Verification items for the finished model (mm, model axes). Face numbers are marked on the shaded views. Round coordinates to 2 decimals unless told otherwise and drop trailing zeros. Write each loop counter-clockwise with the first axis right and the second up, starting at its lowest first coordinate (ties: lowest second). Pieces come first, ordered by that corner, then holes. Notation, with made-up numbers: M 23.25,86 L 34.25,86 A14 ccw 34.25,105 Z; hole C 37.5,23.25 d10. An arc over 180 degrees is marked long. One line per item, written item: value. Start each with the question number.
Item 1: Gauge pin test, flat ends, axial feed: pin 1 (0.9 mm diameter, centred on y = 1.5, z = -32, fed in from +X); pin 2 (1.5 mm diameter, centred on y = 2, z = -28, fed in from -X); pin 3 (1 mm diameter, centred on y = 2.5, z = -56.5, fed in from +X). Record the tip position at first contact, or that the pin passes through.
Item 2: Section check D-D, the plane x = -50.5. Record the cut outline in (y, z), then the cut area to 3 significant figures.
Item 3: Draft check along X on the marked faces 1 and 2. Enter one of: +X half, -X half, draft (parallel to the pull), parting line (faces both ways), or undercut.
Item 4: Section check A-A, the plane z = -54. Record the cut outline in (x, y).
Item 5: Thickness scan on probe 1 along Z at (x, y) = (-4, 2.55); probe 2 along Y at (x, z) = (-83, -25); probe 3 along X at (y, z) = (1.35, -63). Record the ranges inside material, lowest first. Write a range as from..to.
Item 6: Section check B-B, the plane x = -5. Record the cut outline in (y, z).
from build123d import *

# Parameters (mm, degrees)
P_IDAT_VYSUNUT_M1_DEPTH = 3
P_IDAT_VYSUNUT_M2_DEPTH = 2
ZAOBLIT3_R              = 1


with BuildPart() as part:
    # Skica1 → P_idat vysunut_m1 (new body)
    with BuildSketch(Plane(origin=(0, 0, 0), x_dir=(1, 0, 0), z_dir=(0, 1, 0))):
        Polygon((-118.143750166, 15), (-118.143750166, 0), (-102.227105248, 19.278496169), (-95.473037065, 43.348863075), (-82.997228437, 47.003202833), (-48.112980408, 27.430537213), (-19, 0), (0, 0), (0, 15), (9.950504516, 11.37831254), (9.950504516, 24.27831254), (-10.5, 24.27831254), (-10.5, 37.37831254), (0, 33.55662508), (0, 69.224902673), (-39.317553332, 46.524902673), (-78.635106664, 69.224902673), (-118.143185584, 46.414902673), (-118.143185584, 33.5570142), (-107.643750166, 37.378496169), (-107.643750166, 24.278496169), (-128.093750166, 24.278496169), (-128.093750166, 11.378496169), align=None)
    extrude(amount=P_IDAT_VYSUNUT_M1_DEPTH)

    # Skica1_3 → P_idat vysunut_m2 (add)
    with BuildSketch(Plane(origin=(0, 0, 0), x_dir=(1, 0, 0), z_dir=(0, 1, 0))):
        Polygon((-102.227105248, 19.278496169), (-118.143750166, 0), (-19, 0), (-48.112980408, 27.430537213), (-82.997228437, 47.003202833), (-95.473037065, 43.348863075), align=None)
    extrude(amount=P_IDAT_VYSUNUT_M2_DEPTH)

    # Zaoblit3
    zaoblit3_edges = [part.edges().sort_by_distance(p)[0] for p in [
        (-10.5, 1.5, -24.27831254),
        (9.950504516, 1.5, -24.27831254),
        (9.950504516, 1.5, -11.37831254),
        (0, 1.5, -15),
        (-118.143750166, 1.5, -15),
        (-128.093750166, 1.5, -11.378496169),
        (-128.093750166, 1.5, -24.278496169),
        (-107.643750166, 1.5, -24.278496169),
        (-107.643750166, 1.5, -37.378496169),
        (-118.143185584, 1.5, -33.5570142),
        (0, 1.5, -33.55662508),
        (-10.5, 1.5, -37.37831254),
    ]]
    fillet(zaoblit3_edges, radius=ZAOBLIT3_R)


solid = part.part
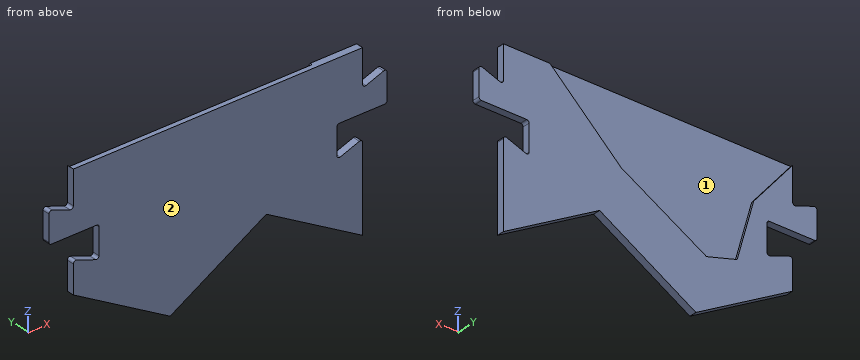
Response values:
1. pin 1: stops at x = -10.5
1. pin 2: stops at x = -107.64
1. pin 3: stops at x = 0
2. outline: M 0,-52.98 L 3,-52.98 L 3,-28.77 L 2,-28.77 L 2,0 L 0,0 Z
2. area: 130 mm2
3. face 1: undercut
3. face 2: draft
4. outline: M -105.01,0 L -52.26,0 L -52.26,3 L -105.01,3 Z; M -26.37,0 L 0,0 L 0,3 L -26.37,3 Z
5. probe 1: z = -66.92..-35.01, -24.28..0
5. probe 2: y = 0..2
5. probe 3: x = -89.42..-67.85, -10.78..0
6. outline: M 0,-66.34 L 3,-66.34 L 3,-35.38 L 0,-35.38 Z; M 0,-24.28 L 3,-24.28 L 3,0 L 0,0 Z
